Can you work these out from the model? Positions are in its coordinate system, mm. A direction names the side the tool comes from. Coordinates: 2 decimals unless noted, no trailing zeros. Write each loop counter-clockwise with the first axis right and the second up, starting at its lowest first coordinate (ties: lowest second). Pieces come first, ordered by that corner, then holes.
```python
from build123d import *

# Parameters (mm, degrees)
SKETCH1_W           = 30
SKETCH1_H           = 13
BOSS_EXTRUDE1_DEPTH = 7.4
BOSS_EXTRUDE2_DEPTH = 14.5
SKETCH3_W           = 10
SKETCH3_H           = 8.5
BOSS_EXTRUDE3_DEPTH = 10
SKETCH5_R           = 1.5
BOSS_EXTRUDE4_DEPTH = 1.5
CUT_EXTRUDE2_DEPTH  = 4
SKETCH7_W           = 10
SKETCH7_H           = 7
BOSS_EXTRUDE5_DEPTH = 8
FILLET1_R           = 1


with BuildPart() as part:
    # Sketch1 → Boss-Extrude1 (new body)
    with BuildSketch(Plane(origin=(0, 0, 0), x_dir=(1, 0, 0), z_dir=(0, 1, 0))):
        Rectangle(SKETCH1_W, SKETCH1_H)
    extrude(amount=BOSS_EXTRUDE1_DEPTH)

    # Sketch2 → Boss-Extrude2 (add)
    with BuildSketch(Plane(origin=(0, 7.4, 0), x_dir=(1, 0, 0), z_dir=(0, 1, 0))):
        with BuildLine():
            Line((-14, 6), (-5, 6))
            ThreePointArc((-5, 6), (-4.292893219, 5.707106781), (-4, 5))
            Line((-4, 5), (-4, -5))
            ThreePointArc((-4, -5), (-4.292893219, -5.707106781), (-5, -6))
            Line((-5, -6), (-14, -6))
            ThreePointArc((-14, -6), (-14.707106781, -5.707106781), (-15, -5))
            Line((-15, -5), (-15, 5))
            ThreePointArc((-15, 5), (-14.707106781, 5.707106781), (-14, 6))
        make_face()
        with BuildLine():
            Line((-13, 5), (-6, 5))
            ThreePointArc((-6, 5), (-5.292893219, 4.707106781), (-5, 4))
            Line((-5, 4), (-5, -4))
            ThreePointArc((-5, -4), (-5.292893219, -4.707106781), (-6, -5))
            Line((-6, -5), (-13, -5))
            ThreePointArc((-13, -5), (-13.707106781, -4.707106781), (-14, -4))
            Line((-14, -4), (-14, 4))
            ThreePointArc((-14, 4), (-13.707106781, 4.707106781), (-13, 5))
        make_face(mode=Mode.SUBTRACT)
        with BuildLine():
            Line((14, 6), (7, 6))
            ThreePointArc((7, 6), (6.292893219, 5.707106781), (6, 5))
            Line((6, 5), (6, -5))
            ThreePointArc((6, -5), (6.292893219, -5.707106781), (7, -6))
            Line((7, -6), (14, -6))
            ThreePointArc((14, -6), (14.707106781, -5.707106781), (15, -5))
            Line((15, -5), (15, 5))
            ThreePointArc((15, 5), (14.707106781, 5.707106781), (14, 6))
        make_face()
        with BuildLine():
            Line((8, -5), (13, -5))
            ThreePointArc((13, -5), (13.707106781, -4.707106781), (14, -4))
            Line((14, -4), (14, 4))
            ThreePointArc((14, 4), (13.707106781, 4.707106781), (13, 5))
            Line((13, 5), (8, 5))
            ThreePointArc((8, 5), (7.292893219, 4.707106781), (7, 4))
            Line((7, 4), (7, -4))
            ThreePointArc((7, -4), (7.292893219, -4.707106781), (8, -5))
        make_face(mode=Mode.SUBTRACT)
    extrude(amount=BOSS_EXTRUDE2_DEPTH)

    # Sketch3 → Boss-Extrude3 (add)
    with BuildSketch(Plane(origin=(0, 7.4, 0), x_dir=(1, 0, 0), z_dir=(0, 1, 0))):
        with Locations((1, -0.15)):
            Rectangle(SKETCH3_W, SKETCH3_H)
    extrude(amount=BOSS_EXTRUDE3_DEPTH)

    # Sketch5 → Boss-Extrude4 (add)
    with BuildSketch(Plane(origin=(0, 0, 0), x_dir=(1, 0, 0), z_dir=(0, 1, 0))):
        with BuildLine():
            Line((-18.5, 4), (18.5, 4))
            ThreePointArc((18.5, 4), (22.5, 0), (18.5, -4))
            Line((18.5, -4), (-18.5, -4))
            ThreePointArc((-18.5, -4), (-22.5, 0), (-18.5, 4))
        make_face()
        with Locations((-18.5, 0)):
            Circle(SKETCH5_R, mode=Mode.SUBTRACT)
        with Locations((18.5, 0)):
            Circle(SKETCH5_R, mode=Mode.SUBTRACT)
    extrude(amount=BOSS_EXTRUDE4_DEPTH)

    # Sketch6 → Cut-Extrude2 (cut)
    with BuildSketch(Plane.XZ):
        Polygon((-14, 5.5), (-5, 5.5), (-5, 6.5), (5, 6.5), (5, 5.5), (14, 5.5), (14, -5.5), (-14, -5.5), align=None)
    extrude(amount=-CUT_EXTRUDE2_DEPTH, mode=Mode.SUBTRACT)

    # Sketch7 → Boss-Extrude5 (add)
    with BuildSketch(Plane.XY.offset(6.5)):
        with Locations((0, 7.5)):
            Rectangle(SKETCH7_W, SKETCH7_H)
    extrude(amount=BOSS_EXTRUDE5_DEPTH)

    # Fillet1
    fillet1_edges = [part.edges().sort_by_distance(p)[0] for p in [
        (-5, 11, 10.5),
        (-5, 4, 10.5),
        (5, 4, 10.5),
        (5, 11, 10.5),
    ]]
    fillet(fillet1_edges, radius=FILLET1_R)


solid = part.part
```
1. I'm going to push flat-ended pins straight in: P1, Ø4, axis at y = 14, z = -2, coming from the -X side; P2, Ø8, axis at x = -10.5, y = 4.5, coming from the +Z side; P3, Ø7.5, axis at x = -10, y = 12.5, coming from the +Z side. Where does each tip first touch, or does it pass through?
2. If we section it at C-C, the plane x = -10: List the corners of the cut face in (y, z) for me, plus the area to 3 significant figures.
3. If we section it at A-A, the plane y = 20.75: Count the separate pieces of the cut face and the enclosed holes in it, plus the area to 3 significant figures.
4. Which directions (+Z, -Z, +X, -X, +Y, -Y) give clear straight access to the entire face, cutting with the end or side of a thin tool? Please do faces 1 (the face through (-4.715, 10.699, 10.556)), 2 (the face through (-13.715, 14.548, -4.699)), 3 (the face through (-10, 15, -6)), 4 (the face through (0, 2, -5.5)).
5. If we section it at D-D, the plane x = -19: List the corners of the cut face in (y, z) for me, plus the area to 3 significant figures.
6. If I drill on L1, parallel to X at y = 0.45, z = 0; L2, parallel to X at y = 17, z = -3.75; L3, parallel to Z at x = 18.5, y = 0.55, over which ranges is the centre line in solid material (lowest first)?
7. We'd pull the mould along X, two halves only. Please class faces 5 (the face through (17, 1, 4)), 6 (the face through (-14.699, 14.548, 5.715)), 7 (the face through (-4, 18, -1)), 8 (the face through (4.699, 10.715, 10.556)): released by +X, released by -X, zero draft, split by the parting line, or undercut.
Answers:
1. P1: stops at x = -15
1. P2: stops at z = 6.5
1. P3: stops at z = 6
2. outline: (0, -6.5) - (7.4, -6.5) - (7.4, -6) - (21.9, -6) - (21.9, -5) - (7.4, -5) - (7.4, 5) - (21.9, 5) - (21.9, 6) - (7.4, 6) - (7.4, 6.5) - (0, 6.5) - (0, 5.5) - (4, 5.5) - (4, -5.5) - (0, -5.5) - close
2. area: 81.2 mm2
3. separate pieces: 2
3. enclosed holes: 2
3. area: 80.0 mm2
4. face 1: +Z, -X, +Y
4. face 2: +Y
4. face 3: -Z, +X, -X, +Y
4. face 4: -Y
5. outline: (0, -3.97) - (1.5, -3.97) - (1.5, -1.41) - (0, -1.41) - close; (0, 1.41) - (1.5, 1.41) - (1.5, 3.97) - (0, 3.97) - close
5. area: 7.66 mm2
6. L1: x = -22.5 to -20, -17 to -14, 14 to 17, 20 to 22.5
6. L2: x = -15 to -14, -5 to 7, 14 to 15
6. L3: z = -4 to -1.5, 1.5 to 4
7. face 5: zero draft
7. face 6: released by -X
7. face 7: undercut
7. face 8: released by +X
